from build123d import *

# Parameters (mm, degrees)
MEMBER_15_15_1_5_1_DEPTH = 135
SKETCH_4_R               = 1.5
CUT_EXTRUDE_1_DEPTH      = 137.037678604


with BuildPart() as part:
    # Sketch1 → Member 15 _15_ 1.5_1 (new body)
    with BuildSketch(Plane(origin=(0, 0, 0), x_dir=(0, 0, -1), z_dir=(1, 0, 0))):
        Polygon((-6, -7.5), (6, -7.5), (7.5, -7.5), (7.5, -6), (7.5, 6), (7.5, 7.5), (6, 7.5), (-6, 7.5), (-7.5, 7.5), (-7.5, 6), (-7.5, -6), (-7.5, -7.5), align=None)
        Polygon((-4, -6), (4, -6), (6, -6), (6, -3.5), (6, 3.5), (6, 6), (3.5, 6), (-3.5, 6), (-5.5, 6), (-5.5, 3.5), (-5.5, -3.5), (-5.5, -6), align=None, mode=Mode.SUBTRACT)
    extrude(amount=MEMBER_15_15_1_5_1_DEPTH)

    # 草图4 → 切除-拉伸1 (cut, through all)
    with BuildSketch(Plane.XZ.offset(7.5)):
        with Locations(Location((38, 0, 0), (0, 0, 270))):
            Circle(SKETCH_4_R)
        with Locations(Location((4, 0, 0), (0, 0, 270))):
            Circle(SKETCH_4_R)
        with Locations(Location((21, 0, 0), (0, 0, 270))):
            Circle(SKETCH_4_R)
    extrude(amount=-CUT_EXTRUDE_1_DEPTH, mode=Mode.SUBTRACT)


solid = part.part
For this review, take the finished solid that the model builds, in its own axes (mm). A direction names the side the tool comes from. Coordinates: 2 decimals unless noted, no trailing zeros. Loops run counter-clockwise (first coordinate to the right, second up) from the corner with the lowest first, then second, coordinate; pieces in that order, holes last. Notation, with made-up numbers: (21, -4.75) - (37, -4.75) arc R25 cw to (37, 12.25) - close; hole circle Ø5 at (66, 58). An arc over 180 degrees is marked (long way). Return JSON: item names as keys, results as strings.
Item 1: Take a section at D-D (x = 95). Give the boundary of the cut face in (y, z).
Determined:
{"outline": "(-7.5, -7.5) - (7.5, -7.5) - (7.5, 7.5) - (-7.5, 7.5) - close; hole (-6, -6) - (6, -6) - (6, 5.5) - (-6, 5.5) - close"}
Item 2: For line 1 (X direction, y = -6.5, z = 0); line 2 (Z direction, x = 118.5, y = -5.25); line 3 (Y direction, x = 23, z = -0.5), list the stretches that pass through material, from the lowest coordinate up.
Determined:
{"line 1": "x = 0 to 2.5, 5.5 to 19.5, 22.5 to 36.5, 39.5 to 135", "line 2": "z = -7.5 to -6, 5.5 to 7.5", "line 3": "y = -7.5 to -6, 6 to 7.5"}
Item 3: Insertion check: pin 1 (3.5 mm diameter, centred on x = 38, z = 0, fed in from -Y). The pin has a flat end and moves straight along its axis. Give the tip position at first contact, or say it passes through.
Determined:
{"pin 1": "stops at y = -7.5"}
Item 4: Take a section at A-A (x = 4). Give the boundary of the cut face in (y, z), then the cut area to 3 significant figures.
Determined:
{"outline": "(-7.5, -7.5) - (7.5, -7.5) - (7.5, -1.5) - (6, -1.5) - (6, -6) - (-6, -6) - (-6, -1.5) - (-7.5, -1.5) - close; (-7.5, 1.5) - (-6, 1.5) - (-6, 5.5) - (6, 5.5) - (6, 1.5) - (7.5, 1.5) - (7.5, 7.5) - (-7.5, 7.5) - close", "area": "78.0 mm2"}
Item 5: Mouldability with a two-part tool opening along Z and no side actions: class faces 3 (the flat face through (67, 0, 5.5)), 4 (the flat face through (0, 0, 7)), 5 (the flat face through (67, 0, -6)), 6 (the flat face through (67, 0, -7.5)) as pulls with the +Z half, pulls with the -Z half, needs draft (parallel to the pull), parting line crosses it, or undercut.
Determined:
{"face 3": "undercut", "face 4": "needs draft", "face 5": "undercut", "face 6": "pulls with the -Z half"}
Item 6: For faces 1 (the flat face through (135, 0, 7)), 2 (the flat face through (67, -6, 0)), list the 3-axis set-ups (+Z, -Z, +X, -X, +Y, -Y) from which the entire face can be reached by the end or side of a thin tool; tool diameter is ignored.
Determined:
{"face 1": "+Z, -Z, +X, +Y, -Y", "face 2": "+X, -X"}
Item 7: Take a section at C-C (y = 1.25). Give the boundary of the cut face in (x, z).
Determined:
{"outline": "(0, -7.5) - (135, -7.5) - (135, -6) - (0, -6) - close; (0, 5.5) - (135, 5.5) - (135, 7.5) - (0, 7.5) - close"}
Item 8: Take a section at B-B (z = 3). Give the boundary of the cut face in (x, y).
Determined:
{"outline": "(0, -7.5) - (135, -7.5) - (135, -6) - (0, -6) - close; (0, 6) - (135, 6) - (135, 7.5) - (0, 7.5) - close"}
